```python
from build123d import *

# Parameters (mm, degrees)
BOSS_EXTRUDE1_DEPTH = 9
BOSS_EXTRUDE2_START = 4
BOSS_EXTRUDE2_DEPTH = 4
CUT_EXTRUDE1_DEPTH  = 4
BOSS_EXTRUDE3_DEPTH = 5
HOLE1_D             = 3.4
HOLE1_DEPTH         = 13.000025
HOLE2_D             = 3.4
HOLE3_D             = 3.4
HOLE4_D             = 26
HOLE5_D             = 3.4
HOLE6_D             = 3.4
HOLE7_D             = 3.4
HOLE8_D             = 3.4
HOLE9_D             = 6.4
HOLE10_D            = 6.4
FILLET1_R           = 5
FILLET2_R           = 5
FILLET3_R           = 5
FILLET4_R           = 5
FILLET5_R           = 7


with BuildPart() as part:
    # Sketch1 → Boss-Extrude1 (new body)
    with BuildSketch(Plane(origin=(0, 0, 0), x_dir=(0, 0, -1), z_dir=(1, 0, 0))):
        with BuildLine():
            Line((-16.707678896, 13.35456662), (-36.5, -12.990381057))
            ThreePointArc((-36.5, -12.990381057), (-39.864082969, -17.679837136), (-38.562263158, -23.302409299))
            Line((-38.562263158, -23.302409299), (-23.47214983, -43.052558883))
            Line((-23.47214983, -43.052558883), (10, -43.052558883))
            Line((10, -43.052558883), (10, -11.451281904))
            Line((10, -11.451281904), (6.09888089, 4.53429444))
            Line((6.09888089, 4.53429444), (-10.960043614, 14.564929128))
            ThreePointArc((-10.960043614, 14.564929128), (-14.030324678, 14.892691596), (-16.707678896, 13.35456662))
        make_face()
    extrude(amount=-BOSS_EXTRUDE1_DEPTH)

    # Sketch2 → Boss-Extrude2 (add)
    with BuildSketch(Plane(origin=(0, 0, 0), x_dir=(0, 0, -1), z_dir=(1, 0, 0)).offset(BOSS_EXTRUDE2_START)):
        with BuildLine():
            Line((-30.213330314, -4.622389094), (-16.707678896, 13.35456662))
            ThreePointArc((-16.707678896, 13.35456662), (-14.030324678, 14.892691596), (-10.960043614, 14.564929128))
            Line((-10.960043614, 14.564929128), (-5.076760086, 11.105562869))
            ThreePointArc((-5.076760086, 11.105562869), (-5.259937554, 7.977270822), (-6.630702447, 5.15933386))
            Line((-6.630702447, 5.15933386), (-16.130702447, -7.34066614))
            ThreePointArc((-16.130702447, -7.34066614), (-24.016200363, -10.355007095), (-30.213330314, -4.622389094))
        make_face()
    extrude(amount=-BOSS_EXTRUDE2_DEPTH)

    # Sketch3 → Cut-Extrude1 (cut)
    with BuildSketch(Plane(origin=(4, 0, 0), x_dir=(0, 0, -1), z_dir=(1, 0, 0))):
        with BuildLine():
            ThreePointArc((-24.560680199, -10.230045092), (-21.25899871, -10.403158596), (-18.1692777, -9.226428797))
            ThreePointArc((-18.1692777, -9.226428797), (-21.620500645, -8.100979585), (-24.560680199, -10.230045092))
        make_face()
    extrude(amount=-CUT_EXTRUDE1_DEPTH, mode=Mode.SUBTRACT)

    # Sketch4 → Boss-Extrude3 (add)
    with BuildSketch(Plane(origin=(-9, 0, 0), x_dir=(0, -1, 0), z_dir=(-1, 0, 0))):
        Polygon((-9.363394526, 33.219335817), (-9.363394526, 19.706149822), (8.623590229, 33.219335817), align=None)
    extrude(amount=-BOSS_EXTRUDE3_DEPTH)

    # Hole1
    with Locations(Plane.ZY.offset(9)):
        with Locations((28.219335817, 4.363394526)):
            Hole(HOLE1_D / 2, depth=HOLE1_DEPTH)

    # Hole2 (through all)
    with Locations(Plane(origin=(4, 0, 0), x_dir=(0, 0, -1), z_dir=(1, 0, 0))):
        with Locations((-13, 10)):
            Hole(HOLE2_D / 2)

    # Hole3 (through all)
    with Locations(Plane(origin=(4, 0, 0), x_dir=(0, 0, -1), z_dir=(1, 0, 0))):
        with Locations((-22.5, -2.5)):
            Hole(HOLE3_D / 2)

    # Hole4 (through all)
    with Locations(Plane(origin=(0, 0, 0), x_dir=(0, 0, -1), z_dir=(1, 0, 0))):
        with Locations((-8, -25.052558883)):
            Hole(HOLE4_D / 2)

    # Hole5 (through all)
    with Locations(Plane(origin=(0, 0, 0), x_dir=(0, 0, -1), z_dir=(1, 0, 0))):
        with Locations((5, -38.052558883)):
            Hole(HOLE5_D / 2)

    # Hole6 (through all)
    with Locations(Plane(origin=(0, 0, 0), x_dir=(0, 0, -1), z_dir=(1, 0, 0))):
        with Locations((-21, -38.052558883)):
            Hole(HOLE6_D / 2)

    # Hole7 (through all)
    with Locations(Plane(origin=(0, 0, 0), x_dir=(0, 0, -1), z_dir=(1, 0, 0))):
        with Locations((-21, -12.052558883)):
            Hole(HOLE7_D / 2)

    # Hole8 (through all)
    with Locations(Plane(origin=(0, 0, 0), x_dir=(0, 0, -1), z_dir=(1, 0, 0))):
        with Locations((5, -12.052558883)):
            Hole(HOLE8_D / 2)

    # Hole9 (through all)
    with Locations(Plane(origin=(0, 0, 0), x_dir=(0, 0, -1), z_dir=(1, 0, 0))):
        with Locations((0, 0)):
            Hole(HOLE9_D / 2)

    # Hole10 (through all)
    with Locations(Plane(origin=(0, 0, 0), x_dir=(0, 0, -1), z_dir=(1, 0, 0))):
        with Locations((-33, -19.052558883)):
            Hole(HOLE10_D / 2)

    # Fillet1
    fillet1_edges = [part.edges().sort_by_distance(p)[0] for p in [
        (-4.5, -43.052558883, -10),
    ]]
    fillet(fillet1_edges, radius=FILLET1_R)

    # Fillet2
    fillet2_edges = [part.edges().sort_by_distance(p)[0] for p in [
        (-4.5, -11.451281904, -10),
    ]]
    fillet(fillet2_edges, radius=FILLET2_R)

    # Fillet3
    fillet3_edges = [part.edges().sort_by_distance(p)[0] for p in [
        (-6.5, 9.363394526, 33.219335817),
    ]]
    fillet(fillet3_edges, radius=FILLET3_R)

    # Fillet4
    fillet4_edges = [part.edges().sort_by_distance(p)[0] for p in [
        (-4.5, -43.052558883, 23.47214983),
    ]]
    fillet(fillet4_edges, radius=FILLET4_R)

    # Fillet5
    fillet5_edges = [part.edges().sort_by_distance(p)[0] for p in [
        (-4.5, 4.53429444, -6.09888089),
    ]]
    fillet(fillet5_edges, radius=FILLET5_R)


solid = part.part
```
Work out the finished part from the listing and answer in its coordinate system (mm). A direction names the side the tool comes from. Coordinates: 2 decimals unless noted, no trailing zeros. Loops run counter-clockwise (first coordinate to the right, second up) from the corner with the lowest first, then second, coordinate; pieces in that order, holes last. Notation, with made-up numbers: (11, 34.25) - (64, 34.25) arc R28 cw to (64, 60.25) - close; hole circle Ø6 at (-23, 52). An arc over 180 degrees is marked (long way). Use a Markdown table: item, result.
Item 1: Find section D-D, the plane y = -2.5. Determine the outline of the cut face in (x, z), and give its area (3 significant figures).
Evaluation:
| item | result |
|---|---|
| outline | (-9, -7.82) - (0, -7.82) - (0, -2) - (-9, -2) - close; (-9, 2) - (0, 2) - (0, 12.45) - (4, 12.45) - (4, 20.8) - (-9, 20.8) - close; (-9, 24.2) - (4, 24.2) - (4, 28.62) - (-4, 28.62) - (-4, 33.22) - (-9, 33.22) - close |
| area | 335 mm2 |
Item 2: Find section A-A, the plane z = 8. Determine the outline of the cut face in (x, y), and give its area (3 significant figures).
Evaluation:
| item | result |
|---|---|
| outline | (-9, -43.05) - (0, -43.05) - (0, -38.05) - (-9, -38.05) - close; (-9, -12.05) - (0, -12.05) - (0, 3.36) - (4, 3.36) - (4, 12.82) - (-9, 12.82) - close |
| area | 307 mm2 |
Item 3: For faces 5 (the flat face through (2.03, -1, 11.31)), 6 (the cylindrical face through (2.028, -8.093, 21.568)), 7 (the cylindrical face through (-2.409, 14.883, 14.073)), determine the directions among +Z, -Z, +X, -X, +Y, -Y from which every point of the face is accessible in a straight line to the end or side of a thin tool.
Evaluation:
| item | result |
|---|---|
| face 5 | -Z, +X, -Y |
| face 6 | +X, -Y |
| face 7 | +X, -X, +Y |
Item 4: Given pin 1 Ø3 at (y, z) = (-38.05, -5) entering from -X; pin 2 Ø2.5 at (x, y) = (-6, -0.5) entering from +Z; pin 3 Ø2.5 at (x, z) = (-6.5, 23) entering from +Y; pin 4 Ø2 at (x, y) = (-1.5, -28) entering from +Z, each flat-ended and moving along its own axis, determine where each tip first touches the part or whether it passes through.
Evaluation:
| item | result |
|---|---|
| pin 1 | passes through |
| pin 2 | stops at z = 33.22 |
| pin 3 | stops at y = 9.36 |
| pin 4 | stops at z = 35.74 |
Item 5: Find section C-C, the plane x = -4.75. State how many separate pieces and enclosed holes the cut face has, and give its area (3 significant figures).
Evaluation:
| item | result |
|---|---|
| separate pieces | 1 |
| enclosed holes | 10 |
| area | 1,610 mm2 |
Item 6: Consider probe 1 along Y at (x, z) = (-4, -0.5); probe 2 along Y at (x, z) = (-5.25, 1); probe 3 along Y at (x, z) = (-8, 26). Determine where each line is inside the solid, lowest interval first. Write a range as from..to.
Evaluation:
| item | result |
|---|---|
| probe 1 | y = -43.05..-34.89, -15.22..-3.16, 3.16..7.83 |
| probe 2 | y = -43.05..-36.01, -14.1..-3.04, 3.04..8.71 |
| probe 3 | y = -39.74..9.36 |
Item 7: Find section B-B, the plane y = -32. Determine the outline of the cut face in (x, z).
Evaluation:
| item | result |
|---|---|
| outline | (-9, -10) - (0, -10) - (0, -2.99) - (-9, -2.99) - close; (-9, 18.99) - (0, 18.99) - (0, 31.92) - (-9, 31.92) - close |
Item 8: The mould has two halves that part along Z. Classify faces 1 (the cylindrical face through (-4.563, 4.145, -5.641)), 2 (the cylindrical face through (-4.56, -12.7, 22.57)), 3 (the flat face through (-4.437, -32.071, 31.863)), 4 (the cylindrical face through (-4.563, -1.947, -2.539)): +Z half, -Z half, draft (parallel to the pull), parting line (faces both ways), or undercut.
Evaluation:
| item | result |
|---|---|
| face 1 | -Z half |
| face 2 | undercut |
| face 3 | +Z half |
| face 4 | undercut |
